```python
from build123d import *

# Parameters (mm, degrees)
CROQUIS2_W              = 50.8
CROQUIS2_H              = 6.31
CROQUIS3_W              = 50.8
CROQUIS3_H              = 6.31
CROQUIS4_W              = 60
CROQUIS4_H              = 53.155
SALIENTE_EXTRUIR1_DEPTH = 6.31
CROQUIS5_W              = 60
CROQUIS5_H              = 6.31
CORTAR_EXTRUIR1_DEPTH   = 6.31
CORTAR_EXTRUIR2_DEPTH   = 634
CROQUIS8_W              = 50.8
CROQUIS8_H              = 6.31
SALIENTE_EXTRUIR2_DEPTH = 63.5
CROQUIS9_R              = 5
CORTAR_EXTRUIR3_DEPTH   = 10
CROQUIS10_W             = 790.847933
CROQUIS10_H             = 6.31
CORTAR_EXTRUIR4_DEPTH   = 286
CROQUIS11_W             = 50.8
CROQUIS11_H             = 6.31
CROQUIS11_W_2           = 210
CORTAR_EXTRUIR5_DEPTH   = 13.11
CROQUIS12_W             = 50.8
CROQUIS12_H             = 6.31
SALIENTE_EXTRUIR3_DEPTH = 6.35
CROQUIS13_W             = 50.8
CROQUIS13_H             = 6.35
CORTAR_EXTRUIR6_DEPTH   = 6.35
CROQUIS14_W             = 260.8
CROQUIS14_H             = 6.31
CORTAR_EXTRUIR7_DEPTH   = 6.31
CROQUIS15_W             = 50.8
CROQUIS15_H             = 6.31
CORTAR_EXTRUIR8_DEPTH   = 6.31
CROQUIS16_W             = 78.776397836
CROQUIS16_H             = 454.479218284
CORTAR_EXTRUIR9_DEPTH   = 128
CROQUIS22_R             = 4.7625
CORTAR_EXTRUIR15_DEPTH  = 33
CROQUIS24_R             = 5.000000022
CORTAR_EXTRUIR18_DEPTH  = 33
CROQUIS25_R             = 4.7625
CORTAR_EXTRUIR19_DEPTH  = 50
CROQUIS26_W             = 50.8
CROQUIS26_H             = 6.31
SALIENTE_EXTRUIR4_DEPTH = 100


with BuildPart() as part:
    # Barrer1: sweep along a curve in space
    with BuildLine() as barrer1_path:
        Line((0, 0, 0), (0, -567.24, 0))
        Line((0, -567.24, 0), (0, -567.24, 336.2))
        Line((0, -567.24, 336.2), (1786.7, -567.24, 336.2))
        Line((1786.7, -567.24, 336.2), (1786.7, -567.24, 693.16))
        Line((1786.7, -567.24, 693.16), (1786.7, -436.23, 693.16))
        Line((1786.7, -436.23, 693.16), (1786.7, -436.23, 1487.162933))
    # Croquis2 → Barrer1 (sweep)
    with BuildSketch(Plane(origin=(0, 0, 0), x_dir=(1, 0, 0), z_dir=(0, 1, 0))):
        Rectangle(CROQUIS2_W, CROQUIS2_H)
        with Locations((210, 0)):
            Rectangle(CROQUIS2_W, CROQUIS2_H)
    sweep(path=barrer1_path.line, transition=Transition.RIGHT)

    # Barrer4: sweep along a curve in space
    with BuildLine() as barrer4_path:
        Line((-0.201028049, -3.155, -3.155), (-0.201028049, -3.155, -207.155))
        Line((-0.201028049, -3.155, -207.155), (-0.201028049, -53.155, -207.155))
    # Croquis3 → Barrer4 (sweep)
    with BuildSketch(Plane(origin=(0, 0, -3.155), x_dir=(-1, 0, 0), z_dir=(0, 0, -1))):
        with Locations((-210, -3.155)):
            Rectangle(CROQUIS3_W, CROQUIS3_H)
        with Locations((0, -3.155)):
            Rectangle(CROQUIS3_W, CROQUIS3_H)
    sweep(path=barrer4_path.line, transition=Transition.RIGHT)

    # Croquis4 → Saliente-Extruir1 (add)
    with BuildSketch(Plane(origin=(0, 0, -210.31), x_dir=(-1, 0, 0), z_dir=(0, 0, -1))):
        with Locations((-154.6, -26.5775)):
            Rectangle(CROQUIS4_W, CROQUIS4_H)
    extrude(amount=-SALIENTE_EXTRUIR1_DEPTH)

    # Croquis5 → Cortar-Extruir1 (cut)
    with BuildSketch(Plane.XY.offset(-204)):
        with Locations((154.6, -3.155)):
            Rectangle(CROQUIS5_W, CROQUIS5_H)
    extrude(amount=-CORTAR_EXTRUIR1_DEPTH, mode=Mode.SUBTRACT)

    # Croquis7 → Cortar-Extruir2 (cut)
    with BuildSketch(Plane(origin=(0, 0, 0), x_dir=(1, 0, 0), z_dir=(0, 1, 0))):
        Polygon((1761.3, -361.6), (2022.1, -361.6), (2022.1, 278.600557529), (-188.115947115, 278.600557529), (-188.115947115, -361.6), align=None)
    extrude(amount=-CORTAR_EXTRUIR2_DEPTH, mode=Mode.SUBTRACT)

    # Croquis8 → Saliente-Extruir2 (add)
    with BuildSketch(Plane(origin=(0, 0, 361.6), x_dir=(-1, 0, 0), z_dir=(0, 0, -1))):
        with Locations((-1786.7, -567.24)):
            Rectangle(CROQUIS8_W, CROQUIS8_H)
    extrude(amount=SALIENTE_EXTRUIR2_DEPTH)

    # Croquis9 → Cortar-Extruir3 (cut)
    with BuildSketch(Plane(origin=(0, -433.075, 0), x_dir=(1, 0, 0), z_dir=(0, 1, 0))):
        with Locations(Location((1786.7, -1454.162933, 0), (0, 0, 270))):
            Circle(CROQUIS9_R)
        with Locations(Location((1786.7, -1234.162933, 0), (0, 0, 270))):
            Circle(CROQUIS9_R)
        with Locations(Location((1996.7, -1234.162933, 0), (0, 0, 270))):
            Circle(CROQUIS9_R)
        with Locations(Location((1996.7, -1454.162933, 0), (0, 0, 270))):
            Circle(CROQUIS9_R)
    extrude(amount=-CORTAR_EXTRUIR3_DEPTH, mode=Mode.SUBTRACT)

    # Croquis10 → Cortar-Extruir4 (cut)
    with BuildSketch(Plane(origin=(2022.1, 0, 0), x_dir=(0, 0, -1), z_dir=(1, 0, 0))):
        with Locations((-1091.7389665, -436.23)):
            Rectangle(CROQUIS10_W, CROQUIS10_H)
    extrude(amount=-CORTAR_EXTRUIR4_DEPTH, mode=Mode.SUBTRACT)

    # Croquis11 → Cortar-Extruir5 (cut)
    with BuildSketch(Plane(origin=(0, -433.075, 0), x_dir=(1, 0, 0), z_dir=(0, 1, 0))):
        with Locations((1996.7, -693.16)):
            Rectangle(CROQUIS11_W, CROQUIS11_H)
        with Locations((1866.3, -693.16)):
            Rectangle(CROQUIS11_W_2, CROQUIS11_H)
    extrude(amount=-CORTAR_EXTRUIR5_DEPTH, mode=Mode.SUBTRACT)

    # Croquis12 → Saliente-Extruir3 (add)
    with BuildSketch(Plane(origin=(0, 0, 361.6), x_dir=(-1, 0, 0), z_dir=(0, 0, -1))):
        with Locations((-1996.7, -567.24)):
            Rectangle(CROQUIS12_W, CROQUIS12_H)
    extrude(amount=SALIENTE_EXTRUIR3_DEPTH)

    # Croquis13 → Cortar-Extruir6 (cut)
    with BuildSketch(Plane(origin=(0, -564.085, 0), x_dir=(1, 0, 0), z_dir=(0, 1, 0))):
        with Locations((1786.7, -301.275)):
            Rectangle(CROQUIS13_W, CROQUIS13_H)
    extrude(amount=-CORTAR_EXTRUIR6_DEPTH, mode=Mode.SUBTRACT)

    # Croquis14 → Cortar-Extruir7 (cut)
    with BuildSketch(Plane(origin=(0, -446.185, 0), x_dir=(1, 0, 0), z_dir=(0, 1, 0))):
        with Locations((1891.7, -693.16)):
            Rectangle(CROQUIS14_W, CROQUIS14_H)
    extrude(amount=-CORTAR_EXTRUIR7_DEPTH, mode=Mode.SUBTRACT)

    # Croquis15 → Cortar-Extruir8 (cut)
    with BuildSketch(Plane(origin=(0, 0, 304.45), x_dir=(-1, 0, 0), z_dir=(0, 0, -1))):
        with Locations((-1786.7, -567.24)):
            Rectangle(CROQUIS15_W, CROQUIS15_H)
    extrude(amount=-CORTAR_EXTRUIR8_DEPTH, mode=Mode.SUBTRACT)

    # Croquis16 → Cortar-Extruir9 (cut)
    with BuildSketch(Plane(origin=(0, -452.495, 0), x_dir=(1, 0, 0), z_dir=(0, 1, 0))):
        with Locations((1993.809618139, -557.908989907)):
            Rectangle(CROQUIS16_W, CROQUIS16_H)
    extrude(amount=-CORTAR_EXTRUIR9_DEPTH, mode=Mode.SUBTRACT)

    # Croquis22 → Cortar-Extruir15 (cut)
    with BuildSketch(Plane(origin=(0, -564.085, 0), x_dir=(1, 0, 0), z_dir=(0, 1, 0))):
        with Locations(Location((1786.7, -551.855, 0), (0, 0, 270))):
            Circle(CROQUIS22_R)
    extrude(amount=-CORTAR_EXTRUIR15_DEPTH, mode=Mode.SUBTRACT)

    # Croquis24 → Cortar-Extruir18 (cut)
    with BuildSketch(Plane(origin=(0, 0, 690.005), x_dir=(-1, 0, 0), z_dir=(0, 0, -1))):
        with Locations((-1786.700000078, -486.49871274)):
            Circle(CROQUIS24_R)
    extrude(amount=-CORTAR_EXTRUIR18_DEPTH, mode=Mode.SUBTRACT)

    # Croquis25 → Cortar-Extruir19 (cut)
    with BuildSketch(Plane(origin=(0, -570.395, 0), x_dir=(-1, 0, 0), z_dir=(0, -1, 0))):
        with Locations(Location((-1799.399999999, -348.862204666, 0), (0, 0, 90))):
            Circle(CROQUIS25_R)
        with Locations(Location((-1773.999999999, -323.462204666, 0), (0, 0, 90))):
            Circle(CROQUIS25_R)
    extrude(amount=-CORTAR_EXTRUIR19_DEPTH, mode=Mode.SUBTRACT)

    # Croquis26 → Saliente-Extruir4 (add)
    with BuildSketch(Plane(origin=(0, -452.495, 0), x_dir=(1, 0, 0), z_dir=(0, 1, 0))):
        with Locations((1786.7, -693.16)):
            Rectangle(CROQUIS26_W, CROQUIS26_H)
    extrude(amount=SALIENTE_EXTRUIR4_DEPTH)


solid = part.part
```
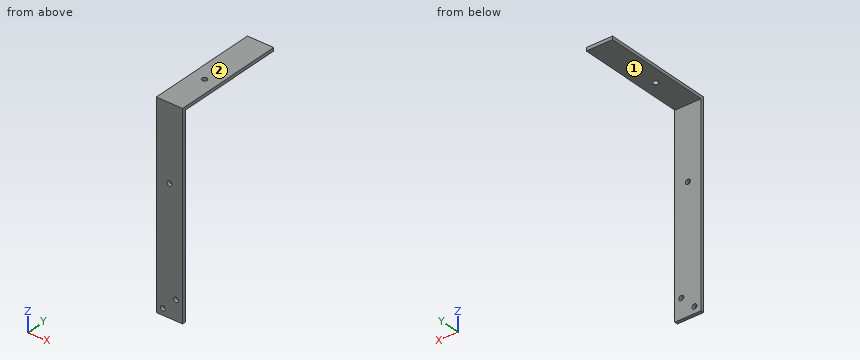
Check sheet for the modelled part. Datum: model origin and axes. Units: mm. Face numbers are marked on the shaded views. A direction names the side the tool comes from. Coordinates: 2 decimals unless noted, no trailing zeros. Loops run counter-clockwise (first coordinate to the right, second up) from the corner with the lowest first, then second, coordinate; pieces in that order, holes last.
1) Material ranges on probe 1 along Z at (x, y) = (1774, -567.5) (3 decimals); probe 2 along Z at (x, y) = (1786.7, -568.25) (1 decimal); probe 3 along Y at (x, z) = (1786, 691) (3 decimals), recorded low to high.
2) Sectioned sample at B-B (z = 537.5). Record the boundary of the cut face in (x, y) (3 decimals).
3) Gauge pin test, flat ends, axial feed: pin 1 (11 mm diameter, centred on x = 1786.7, z = 551.855, fed in from -Y) (3 decimals); pin 2 (10 mm diameter, centred on x = 1768, z = 563, fed in from +Y) (3 decimals); pin 3 (6 mm diameter, centred on x = 1786.7, y = -486.5, fed in from +Z). Record the tip position at first contact, or that the pin passes through.
4) Sectioned sample at A-A (x = 1774). Record the boundary of the cut face in (y, z) (3 decimals).
5) Access from +Z, -Z, +X, -X, +Y, -Y to the whole of each face (thin tool, end or side, straight path). Record for the marked faces 1 and 2.
6) Sectioned sample at C-C (y = -368). Record the boundary of the cut face in (x, z) (3 decimals).
Check sheet entries:
1. probe 1: z = 310.76 to 318.7, 328.225 to 696.315
1. probe 2: z = 310.8 to 547.1, 556.6 to 696.3
1. probe 3: y = -570.395 to -491.449, -481.548 to -352.495
2. outline: (1761.3, -570.395) - (1812.1, -570.395) - (1812.1, -564.085) - (1761.3, -564.085) - close
3. pin 1: stops at y = -570.395
3. pin 2: stops at y = -564.085
3. pin 3: passes through
4. outline: (-570.395, 310.76) - (-564.085, 310.76) - (-564.085, 318.7) - (-570.395, 318.7) - close; (-570.395, 328.225) - (-564.085, 328.225) - (-564.085, 690.005) - (-352.495, 690.005) - (-352.495, 696.315) - (-570.395, 696.315) - close
5. face 1: -Z, +X, -X, +Y
5. face 2: +Z, +X, -X, +Y, -Y
6. outline: (1761.3, 690.005) - (1812.1, 690.005) - (1812.1, 696.315) - (1761.3, 696.315) - close
